Autodesk Inventor part; units mm, degrees
ref_plane "YZ Plane" through (0, 0, 0) normal (1, 0, 0) x (0, 1, 0)
ref_plane "XZ Plane" through (0, 0, 0) normal (0, 1, 0) x (-1, 0, 0)
ref_plane "XY Plane" through (0, 0, 0) normal (0, 0, 1) x (1, 0, 0)
sketch "Sketch1" plane through (0, 0, 0) normal (0, 0, 1) x (1, 0, 0)
  circle A0 centre (0, 0) radius 3
  dimension "Diameter" = 6
extrude "Extrusion1" add sketch "Sketch1" along normal blind 70
sketch "Sketch2" plane through (0, 0, 70) normal (0, 0, 1) x (1, 0, 0)
  circle A0 centre (0, 0) radius 3
  circle A1 centre (0, 0) radius 5
  dimension "Head_Diameter" = 10
extrude "Extrusion2" add sketch "Sketch2" along normal blind 6 contours A0 | A1
sketch "Sketch3" plane through (0, 0, 76) normal (0, 0, 1) x (1, 0, 0)
  circle A0 centre (0, 0) radius 5
  circle A1 centre (0, 0) radius 2.8868 construction
  line L0 (0, 2.8868) -> (2.5, 1.4434)
  line L1 (2.5, -1.4434) -> (2.5, 1.4434)
  line L2 (0, 2.8868) -> (-2.5, 1.4434)
  line L3 (-2.5, -1.4434) -> (-2.5, 1.4434)
  line L4 (-2.5, -1.4434) -> (0, -2.8868)
  line L5 (2.5, -1.4434) -> (0, -2.8868)
  dimension "Hex_Width" = 5
extrude "Extrusion3" cut sketch "Sketch3" against normal blind 3 contours L0 L1 L5 L4 L3 L2
thread "Thread1"
chamfer "Chamfer1" distance 0.6 angle 45 2 edges at (-5, 0, 76) (-3, 0, 0)
equation "\"d9\" = ThreadLength"
equation "\"d12\" = Chamfer"
equation "\"ThreadLength\" = 24"
properties part number "SCREW, SOCKET HD, P, 12.9, M6X1.0X70MM"
Verification items for the finished model (mm, model axes). A direction names the side the tool comes from. Round coordinates to 2 decimals unless told otherwise and drop trailing zeros. Loops run counter-clockwise (first coordinate to the right, second up) from the corner with the lowest first, then second, coordinate; pieces in that order, holes last. Notation, with made-up numbers: (32.25, 36.25) - (90.25, 36.25) arc R26 ccw to (90.25, 50.25) - close; hole circle Ø5 at (-33.5, 38). An arc over 180 degrees is marked (long way). Use one line per item in the form item = value.
1. Scan lines: probe 1 along Z at (x, y) = (1.75, 1); probe 2 along Z at (x, y) = (3.25, 2); probe 3 along X at (y, z) = (-1.75, 43). Record each from-to range of solid material in increasing order.
A:
probe_1 = 0 to 73
probe_2 = 70 to 76
probe_3 = -2.44 to 2.44
2. Draft check along X on faces 1 (the flat face through (2.5, 0, 75)), 2 (the flat face through (2, -2, 76)), 3 (the cylindrical face through (-3, 0, 35)). Enter one of: pulls with the +X half, pulls with the -X half, needs draft (parallel to the pull), parting line crosses it, or undercut.
A:
face_1 = undercut
face_2 = needs draft
face_3 = parting line crosses it
3. Section check B-B on z = 16. Record the cut outline in (x, y), and give its area (3 significant figures).
A:
outline = circle Ø6 at (0, 0)
area = 28.3 mm²
4. Section check A-A on y = 0. Record the cut outline in (x, z).
A:
outline = (-5, 70) - (-3, 70) - (-3, 0.6) - (-2.4, 0) - (2.4, 0) - (3, 0.6) - (3, 70) - (5, 70) - (5, 75.4) - (4.4, 76) - (2.5, 76) - (2.5, 73) - (-2.5, 73) - (-2.5, 76) - (-4.4, 76) - (-5, 75.4) - close
5. Access from +Z, -Z, +X, -X, +Y, -Y to the whole of each face (thin tool, end or side, straight path). Record for faces 4 (the flat face through (-1.233, 2.175, 74.521)), 5 (the cylindrical face through (-1.08, 4.88, 72.66)), 6 (the flat face through (3.3, 0.1, 70)).
A:
face_4 = +Z
face_5 = +Z, -Z
face_6 = -Z
6. Gauge pin test, flat ends, axial feed: pin 1 Ø6 at (y, z) = (-1, 41.5) entering from -X; pin 2 Ø3 at (x, z) = (-2, 44.5) entering from -Y; pin 3 Ø1.5 at (x, z) = (3.5, 47) entering from +Y. Record the tip position at first contact, or that the pin passes through.
A:
pin_1 = -3
pin_2 = -2.96
pin_3 = 1.2
